Source: CAD feature listing. Evaluate the final solid. Frame: model axes, mm. A direction names the side the tool comes from. Round coordinates to 2 decimals unless told otherwise and drop trailing zeros. Loops run counter-clockwise (first coordinate to the right, second up) from the corner with the lowest first, then second, coordinate; pieces in that order, holes last. Notation, with made-up numbers: M 18.25,86.25 L 71.25,86.25 A17 cw 71.25,115.25 Z; hole C 73,-17.75 d8. An arc over 180 degrees is marked long. Answer as a JSON object with one key per item and string values.
from build123d import *

# Parameters (mm, degrees)
F0_W     = 406.4
F0_H     = 406.4
F0_W_2   = 393.7
F0_H_2   = 393.7
F1_DEPTH = 406.4
F2_W     = 406.4
F2_H     = 406.4
F2_R     = 3.175
F2_R_2   = 2.032
F3_DEPTH = 406.4


with BuildPart() as f1:
    # F0 (on Right) → F1 (new body)
    with BuildSketch(Plane.YZ):
        Rectangle(F0_W, F0_H)
        Rectangle(F0_W_2, F0_H_2, mode=Mode.SUBTRACT)
    extrude(amount=F1_DEPTH)

    # F2 (on face) → F3 (intersect)
    with BuildSketch(Plane.XZ.offset(203.2)):
        with Locations((203.2, 0)):
            Rectangle(F2_W, F2_H)
        with Locations((96.52, -184.072345)):
            Circle(F2_R, mode=Mode.SUBTRACT)
        with Locations((149.86, -184.072345)):
            Circle(F2_R, mode=Mode.SUBTRACT)
        with Locations((96.52, -6.35)):
            Circle(F2_R, mode=Mode.SUBTRACT)
        with Locations((256.54, -184.072345)):
            Circle(F2_R, mode=Mode.SUBTRACT)
        with Locations((203.2, 0)):
            Circle(F2_R_2, mode=Mode.SUBTRACT)
        with Locations((149.86, 71.191654)):
            Circle(F2_R, mode=Mode.SUBTRACT)
        with Locations((256.54, 71.191654)):
            Circle(F2_R, mode=Mode.SUBTRACT)
    extrude(amount=-F3_DEPTH, mode=Mode.INTERSECT)


solid = f1.part
Item 1: Section A-A on y = -64. Return the cut outline in (x, z).
Answer sheet:
{"outline": "M 0,-203.2 L 406.4,-203.2 L 406.4,-196.85 L 0,-196.85 Z; M 0,196.85 L 406.4,196.85 L 406.4,203.2 L 0,203.2 Z"}
Item 2: Pull-direction query (Y, two-part tool) for faces 3 (the flat face through (200, -3, -203.2)), 4 (the flat face through (200, -196.85, -3)), 5 (the flat face through (200, -203.2, -3)); classes: pulls with the +Y half, pulls with the -Y half, needs draft (parallel to the pull), parting line crosses it, or undercut.
Answer sheet:
{"face 3": "needs draft", "face 4": "undercut", "face 5": "pulls with the -Y half"}
Item 3: Line query: probe 1 along Z at (x, y) = (149, 200); probe 2 along Z at (x, y) = (256.54, -199); probe 3 along Y at (x, z) = (78.5, 98). Output: solid intervals per line, ascending. Write a range as from..to.
Answer sheet:
{"probe 1": "z = -203.2..-187.13, -181.02..68.14, 74.25..203.2", "probe 2": "z = -203.2..-187.25, -180.9..68.02, 74.37..203.2", "probe 3": "y = -203.2..-196.85, 196.85..203.2"}
Item 4: Contact query for a flat-ended pin moving along its axis: pin 1 Ø7.5 at (x, z) = (96.52, -6.35) entering from +Y. Output: stop coordinate, or through.
Answer sheet:
{"pin 1": "stops at y = 203.2"}
Item 5: Section C-C on x = 212. Return the cut outline in (y, z), then the cut area to 3 significant figures.
Answer sheet:
{"outline": "M -203.2,-203.2 L 203.2,-203.2 L 203.2,203.2 L -203.2,203.2 Z; hole M -196.85,-196.85 L 196.85,-196.85 L 196.85,196.85 L -196.85,196.85 Z", "area": "10,200 mm²"}
Item 6: Access query for faces 1 (the flat face through (200, 203.2, -3)), 2 (the flat face through (200, 196.85, -3)). Directions: +Z, -Z, +X, -X, +Y, -Y. A direction counts if a zero-diameter tool reaches every point of the face in a straight line with its end or side. Return the directions, or none.
Answer sheet:
{"face 1": "+Z, -Z, +X, -X, +Y", "face 2": "+X, -X"}
